```python
from build123d import *

# Parameters (mm, degrees)
SKETCH_W     = 40
SKETCH_H     = 40
PAD_DEPTH    = 12
SKETCH001_R  = 9
PAD001_DEPTH = 25
SKETCH002_R  = 4.5
PAD002_DEPTH = 15


with BuildPart() as part:
    # Sketch → Pad (new body)
    with BuildSketch(Plane.XY):
        with Locations((20, 20)):
            Rectangle(SKETCH_W, SKETCH_H)
    extrude(amount=PAD_DEPTH)

    # Sketch001 → Pad001 (join)
    with BuildSketch(Plane.XY):
        with Locations((15, 10)):
            Circle(SKETCH001_R)
    extrude(amount=PAD001_DEPTH)

    # Sketch002 → Pad002 (join, symmetric)
    with BuildSketch(Plane.YZ):
        with Locations((30, 8)):
            Circle(SKETCH002_R)
    extrude(amount=PAD002_DEPTH, both=True)


solid = part.part
```
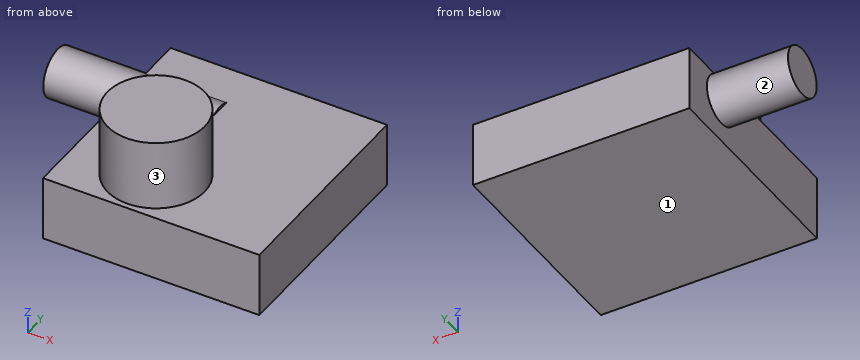
For this review, take the finished solid that the model builds, in its own axes (mm). Face numbers are marked on the shaded views. A direction names the side the tool comes from. Round coordinates to 2 decimals unless told otherwise and drop trailing zeros. Write each loop counter-clockwise with the first axis right and the second up, starting at its lowest first coordinate (ties: lowest second). Pieces come first, ordered by that corner, then holes. Notation, with made-up numbers: (74, -30) -> (111, -30) arc R4 cw to (111, -24) -> close; hole circle Ø9 at (9, -37). An arc over 180 degrees is marked (long way). One line per question, with ' | ' between items. Start each with the question number.
1) Add section C-C (z = 17.75). Write out the cut boundary in (x, y), and give its area (3 significant figures).
2) Machinability: for the marked faces 1, 2 and 3, which of the approach directions +Z, -Z, +X, -X, +Y, -Y give a long, thin tool a straight path to every point of the face, cutting with its end or side? Answer none if there is none.
3) Wall thickness on line 1 along Z through (x, y) = (9, 21.5); line 2 along X through (y, z) = (10, 3.25); line 3 along X through (y, z) = (15, 23): over which ranges is each line inside the solid? List them lowest first.
4) Add section A-A (y = 30). Write out the cut boundary in (x, z).
5) Add section B-B (x = 23). Write out the cut boundary in (y, z), and give its area (3 significant figures).
6) Add section D-D (x = 11.5). Write out the cut boundary in (y, z), and give its area (3 significant figures).
7) For pin 1 Ø6 at (x, y) = (33.5, 14) entering from +Z; pin 2 Ø2 at (x, z) = (11.5, 13.5) entering from -Y; pin 3 Ø9.5 at (y, z) = (12.5, 5.5) entering from -X, all flat-tipped, find the tip position at first contact; note any pin that passes through.
Reported:
1) outline: circle Ø18 at (15, 10) | area: 254 mm²
2) face 1: -Z, +X, -X, +Y, -Y | face 2: -X | face 3: +Z
3) line 1: z = 0 to 12 | line 2: x = 0 to 40 | line 3: x = 7.52 to 22.48
4) outline: (-15, 3.5) -> (0, 3.5) -> (0, 0) -> (40, 0) -> (40, 12) -> (15, 12) -> (15, 12.5) -> (-15, 12.5) -> close
5) outline: (0, 0) -> (40, 0) -> (40, 12) -> (14.12, 12) -> (14.12, 25) -> (5.88, 25) -> (5.88, 12) -> (0, 12) -> close | area: 587 mm²
6) outline: (0, 0) -> (40, 0) -> (40, 12) -> (32.06, 12) arc R4.5 ccw to (27.94, 12) -> (18.29, 12) -> (18.29, 25) -> (1.71, 25) -> (1.71, 12) -> (0, 12) -> close | area: 697 mm²
7) pin 1: stops at z = 12 | pin 2: stops at y = 1.35 | pin 3: stops at x = 0
